Input: part model. Units: mm. Frame: model coordinates. A direction names the side the tool comes from. Round coordinates to 2 decimals unless told otherwise and drop trailing zeros. Write each loop counter-clockwise with the first axis right and the second up, starting at its lowest first coordinate (ties: lowest second). Pieces come first, ordered by that corner, then holes. Notation, with made-up numbers: (-9.75, 7.25) -> (41.25, 7.25) arc R11 cw to (41.25, 15.25) -> close; hole circle Ø10 at (-22.75, 81). An arc over 180 degrees is marked (long way). Use CSV: the item, a comma, the result in double quotes.
```python
from build123d import *

# Parameters (mm, degrees)
F0_W     = 50
F0_H     = 38
F1_DEPTH = 38
F2_W     = 50
F2_H     = 20
F3_DEPTH = 5
F4_R     = 1.25
F5_DEPTH = 25
F7_DEPTH = 5


with BuildPart() as f1:
    # F0 (on Top) → F1 (new body)
    with BuildSketch(Plane.XY):
        with Locations((25, -19)):
            Rectangle(F0_W, F0_H)
    extrude(amount=F1_DEPTH)

    # F2 (on face) → F3 (cut)
    with BuildSketch(Plane.XY.offset(38)):
        with Locations((25, -25)):
            Rectangle(F2_W, F2_H)
    extrude(amount=-F3_DEPTH, mode=Mode.SUBTRACT)

    # F4 (on face) → F5 (cut)
    with BuildSketch(Plane.XZ.offset(15)):
        with Locations((10, 35.5)):
            Circle(F4_R)
        with Locations((40, 35.5)):
            Circle(F4_R)
    extrude(amount=-F5_DEPTH, mode=Mode.SUBTRACT)

    # F6 (on face) → F7 (cut)
    with BuildSketch(Plane.XZ.offset(38)):
        Polygon((11.224955, 38), (8.775045, 38), (9.125, 34), (10.875, 34), align=None)
        Polygon((41.224955, 38), (38.775045, 38), (39.125, 34), (40.875, 34), align=None)
    extrude(amount=-F7_DEPTH, mode=Mode.SUBTRACT)


solid = f1.part
```
Item 1: Line query: line 1 (Z direction, x = 10, y = -5); line 2 (X direction, y = -11, z = 35); line 3 (X direction, y = -35.5, z = 34.5). Output: solid intervals per line, ascending.
Worked answers:
line 1,"z = 0 to 34.25, 36.75 to 38"
line 2,"x = 0 to 8.85, 11.15 to 38.85, 41.15 to 50"
line 3,"x = 0 to 9.08, 10.92 to 39.08, 40.92 to 50"
Item 2: Section query D-D on y = -18. Return the cut outline in (x, z), plus the area to 3 significant figures.
Worked answers:
outline,"(0, 0) -> (50, 0) -> (50, 33) -> (0, 33) -> close"
area,"1,650 mm²"
Item 3: Section query B-B on z = 35.5. Return the cut outline in (x, y), plus the area to 3 significant figures.
Worked answers:
outline,"(0, -38) -> (8.99, -38) -> (8.99, -35) -> (0, -35) -> close; (0, -15) -> (8.75, -15) -> (8.75, 0) -> (0, 0) -> close; (11.01, -38) -> (38.99, -38) -> (38.99, -35) -> (11.01, -35) -> close; (11.25, -15) -> (38.75, -15) -> (38.75, 0) -> (11.25, 0) -> close; (41.01, -38) -> (50, -38) -> (50, -35) -> (41.01, -35) -> close; (41.25, -15) -> (50, -15) -> (50, 0) -> (41.25, 0) -> close"
area,"813 mm²"
Item 4: Section query C-C on x = 15. Return the cut outline in (y, z), plus the area to 3 significant figures.
Worked answers:
outline,"(-38, 0) -> (0, 0) -> (0, 38) -> (-15, 38) -> (-15, 33) -> (-35, 33) -> (-35, 38) -> (-38, 38) -> close"
area,"1,340 mm²"
Item 5: Set-up query: faces 5 (the face through (25, -35, 36)), 6 (the face through (39.01, -7.6, 34.74)), 7 (the face through (41.048, -36.521, 35.972)). Return all of +Z, -Z, +X, -X, +Y, -Y with unobstructed straight access to the full face (end or side cutting, diameter ignored); none if empty.
Worked answers:
face 5,"+Z, +X, -X"
face 6,"+Y"
face 7,"+Z, -Y"
Item 6: Pull-direction query (Y, two-part tool) for faces 1 (the face through (25, -15, 36)), 2 (the face through (9.01, -7.6, 34.74)), 3 (the face through (25, 0, 19)), 4 (the face through (25, -38, 19)); classes: +Y half, -Y half, draft (parallel to the pull), parting line (faces both ways), or undercut.
Worked answers:
face 1,"undercut"
face 2,"draft"
face 3,"+Y half"
face 4,"-Y half"
Item 7: Section query A-A on x = 10. Return the cut outline in (y, z).
Worked answers:
outline,"(-38, 0) -> (0, 0) -> (0, 34.25) -> (-15, 34.25) -> (-15, 33) -> (-35, 33) -> (-35, 34) -> (-38, 34) -> close; (-15, 36.75) -> (0, 36.75) -> (0, 38) -> (-15, 38) -> close"
Item 8: First-contact query: pin 1 Ø0.5 at (x, y) = (9.5, -36) entering from +Z. Flat tip, straight axial feed; report the tip coordinate or a pass-through.
Worked answers:
pin 1,"stops at z = 34"
